Build history of the part. All positions in model axes, mm. A direction names the side the tool comes from. Give positions to 0.01 mm unless a question says otherwise; leave off trailing zeros. Order: outer loops, then holes, each group sorted by start corner. A loop starts at its lowest first (then second) coordinate and runs counter-clockwise, first axis right, second up. Notation, with made-up numbers: (51.5, 40) -> (82.5, 40) arc R21 cw to (82.5, 53) -> close; hole circle Ø3 at (-19, 76.25). An arc over 180 degrees is marked (long way). One line per item, written item: value. Start each with the question number.
(1) Saw through at B-B on y = 74.5. Give the cut face in (x, z).
(2) Which spindle directions (+Z, -Z, +X, -X, +Y, -Y) get a long thin tool onto all of the face, cutting with end or side? Do faces 1 (the flat face through (5, 90, 25)), 2 (the flat face through (60.07, 83.8, 38.87)), 3 (the flat face through (127.535, 29.615, 24.65)), 4 (the flat face through (73.033, 50.897, 35.14)), 5 (the flat face through (88, 32, 0)). Say none if no direction does.
(3) Two-plate mould, pull along Y, no slides. Class faces 6 (the flat face through (60.07, 83.8, 11.13)), 7 (the flat face through (129.93, 29.78, 24.65)), 8 (the flat face through (36, 87.5, 25)), 9 (the flat face through (21, 90, 37.5)): +Y half, -Y half, draft (parallel to the pull), parting line (faces both ways), or undercut.
(4) Saw through at D-D on z = 17.5. Count the separate pieces of the cut face and the enclosed holes in it, plus the area to 3 significant figures.
(5) Saw through at C-C on y = 30. Give the cut face in (x, z).
(6) Pin check, flat tips, straight feed: pin 1 (4 mm diameter, centred on x = 41, z = 9, fed in from -Y); pin 2 (5 mm diameter, centred on x = 61.5, z = 21, fed in from -Y); pin 3 (5.5 mm diameter, centred on x = 15, z = 25, fed in from -Y); pin 4 (6 mm diameter, centred on y = 46.5, z = 27.5, fed in from +X). Stop position of each tip, or through.
(7) Saw through at A-A on x = 30. Give the cut face in (y, z).
(8) Probe line 1 (Z direction, x = 15, y = 89.5); line 2 (Y direction, x = 12, z = 19.5); line 3 (Y direction, x = 98, z = 42). List the from-to ranges inside material, lowest first.
```python
from build123d import *

# Parameters (mm, degrees)
PAD_DEPTH       = 50
POCKET_DEPTH    = 10
POCKET001_DEPTH = 5
POCKET002_DEPTH = 5
POCKET003_DEPTH = 86.7059680197
SKETCH001_R     = 3
HOLE_DEPTH      = 92.501


with BuildPart() as part:
    # Sketch → Pad (new body)
    with BuildSketch(Plane.XY):
        Polygon((5, 92.5), (65, 92.5), (65, 67.5), (105, 16.2652461702), (130, 16.2652461702), (130, 23.7652461702), (125, 35.6301629012), (135, 23.7652461702), (135, 3.4565577128), (105, 3.4565577128), (55, 67.5), (55, 87.5), (5, 87.5), align=None)
    extrude(amount=PAD_DEPTH)

    # Sketch005 → Pocket (cut)
    with BuildSketch(Plane.YZ.offset(65)):
        Polygon((72.5, 47.5), (87.5, 47.5), (80, 30), align=None)
        Polygon((80, 20), (72.5, 2.5), (87.5, 2.5), align=None)
        Polygon((71, 40), (77.5, 25), (71, 10), align=None)
        Polygon((82.5, 25), (89, 40), (89, 10), align=None)
    extrude(amount=-POCKET_DEPTH, mode=Mode.SUBTRACT)

    # Sketch002 → Pocket001 (cut)
    with BuildSketch(Plane(origin=(0, 92.5, 0), x_dir=(-1, 0, 0), z_dir=(0, 1, 0))):
        Polygon((-52.5, 50), (-37.5, 37.5), (-5, 37.5), (-5, 50), align=None)
    extrude(amount=-POCKET001_DEPTH, mode=Mode.SUBTRACT)

    # Sketch003 → Pocket002 (cut)
    with BuildSketch(Plane(origin=(0, 92.5, 0), x_dir=(-1, 0, 0), z_dir=(0, 1, 0))):
        Polygon((-52.5, 0), (-37.5, 12.500000002), (-5, 12.5), (-5, 0), align=None)
    extrude(amount=-POCKET002_DEPTH, mode=Mode.SUBTRACT)

    # Sketch008 (on Face23 of Pocket002) → Pocket003 (cut, through all)
    with BuildSketch(Plane(origin=(73.1263515599, 57.0912094574, 0), x_dir=(-0.6153846154, 0.788226982, 0), z_dir=(0.788226982, 0.6153846154, 0))):
        Polygon((7.5, 5), (7.5, 45), (-17.5, 25), align=None)
        Polygon((-47.5, 5), (-47.5, 45), (-22.5, 25), align=None)
        Polygon((-0.005547, 45.032113), (-40.0240908379, 44.9926101173), (-20, 30), align=None)
        Polygon((-20, 20), (0, 4.9752679886), (-40.0185556925, 5), align=None)
    extrude(amount=-POCKET003_DEPTH, mode=Mode.SUBTRACT)

    # Sketch001 → Hole (cut, through all)
    with BuildSketch(Plane.XZ):
        with Locations((15, 25)):
            Circle(SKETCH001_R)
        with Locations((30, 25)):
            Circle(SKETCH001_R)
    extrude(amount=-HOLE_DEPTH, mode=Mode.SUBTRACT)


solid = part.part
```
Results below:
1. outline: (55, 0) -> (65, 0) -> (65, 2.5) -> (55, 2.5) -> close; (55, 7.17) -> (65, 7.17) -> (65, 18.08) -> (55, 18.08) -> close; (55, 31.92) -> (65, 31.92) -> (65, 42.83) -> (55, 42.83) -> close; (55, 47.5) -> (65, 47.5) -> (65, 50) -> (55, 50) -> close
2. face 1: +Z, -Z, -X, +Y, -Y
2. face 2: +X, -X
2. face 3: +Z, -Z
2. face 4: none
2. face 5: -Z, +X, -X, +Y, -Y
3. face 6: undercut
3. face 7: +Y half
3. face 8: -Y half
3. face 9: draft
4. separate pieces: 7
4. enclosed holes: 0
4. area: 1,140 mm²
5. outline: (84.28, 0) -> (94.28, 0) -> (94.28, 5) -> (84.28, 4.99) -> close; (84.28, 13.84) -> (94.28, 9.23) -> (94.28, 15.5) -> (84.28, 20.43) -> close; (84.28, 29.57) -> (94.28, 34.5) -> (94.28, 40.76) -> (84.28, 36.15) -> close; (84.28, 45) -> (94.28, 45) -> (94.28, 50) -> (84.28, 50) -> close; (127.37, 0) -> (129.75, 0) -> (129.75, 50) -> (127.37, 50) -> close
6. pin 1: stops at y = 87.5
6. pin 2: stops at y = 58.15
6. pin 3: passes through
6. pin 4: stops at x = 83.74
7. outline: (87.5, 12.5) -> (92.5, 12.5) -> (92.5, 22) -> (87.5, 22) -> close; (87.5, 28) -> (92.5, 28) -> (92.5, 37.5) -> (87.5, 37.5) -> close
8. line 1: z = 12.5 to 22, 28 to 37.5
8. line 2: y = 87.5 to 92.5
8. line 3: y = 12.42 to 16.25, 21.01 to 25.23
